Autodesk Inventor part; units mm, degrees
ref_plane "Work Plane1" through (29, 0, 0) normal (0, -1, 0) x (1, 0, 0)
ref_plane "YZ Plane" through (0, 0, 0) normal (1, 0, 0) x (0, 1, 0)
ref_plane "XZ Plane" through (0, 0, 0) normal (0, 1, 0) x (-1, 0, 0)
sketch "Sketch1" plane through (0, 0, 0) normal (0, 0, 1) x (1, 0, 0)
  line L0 (-2.6667, 0) -> (20, 0)
  line L1 (20, 0) -> (20, 6)
  line L2 (20, 6) -> (4.375, 6)
  line L3 (4.375, 6) -> (3.3014, 6)
  line L4 (3.3014, 6) -> (0, 6)
  line L5 (0, 6) -> (0, 9)
  line L6 (0, 9) -> (-12, 9)
  line L7 (-12, 9) -> (-12, 5.7735)
  line L8 (-12, 5.7735) -> (-6, 5.7735)
  line L9 (-6, 5.7735) -> (-2.6667, 0)
  line L10 (-18.4, 0) -> (26.4, 0)
  line L11 (0, -1.8) -> (0, 10.8)
  line L12 (4.375, 6) -> (0, 6) construction
  dimension "d1" = 15.625
  dimension "d2" = 1.0736
  dimension "d3" = 12
  dimension "d4" = 6
  dimension "d5" = 60
  dimension "d6" = 12
  dimension "d7" = 12
  dimension "d8" = 11.547
  dimension "d9" = 18
  dimension "d26" = 20
revolve "Body" add sketch "Sketch1" angle 360 about axis through (-2.6667, 0, 0) along (1, 0, 0)
sketch "Sketch2" plane through (-12, 0, 0) normal (-1, 0, 0) x (0, 0, 1)
  circle A0 centre (0, 0) radius 5.7735
  line L0 (0, -12.6) -> (0, 12.6)
  line L1 (-12.6, 0) -> (12.6, 0)
  line L2 (5.7735, 0) -> (2.8868, -5)
  line L3 (2.8868, -5) -> (-2.8868, -5)
  line L4 (-2.8868, -5) -> (-5.7735, 0)
  line L5 (-5.7735, 0) -> (-2.8868, 5)
  line L6 (-2.8868, 5) -> (2.8868, 5)
  line L7 (2.8868, 5) -> (5.7735, 0)
extrude "Slot" add sketch "Sketch2" against normal up to next contours L7 A0 | A0 L2 | L6 L0 A0 | A0 L0 L3 | L0 L6 A0 | A0 L3 L0 | L4 A0 | A0 L5
fillet "Fillet1" radius 1.2 1 edges at (-12, -9, 0)
thread "Thread"
chamfer "Chamfer1" distance 1.0735 distance2 1.0735 1 edges at (20, -6, 0) measured on face at (20, -3.0269, -1.5886)
ref_plane "Work Plane1" through (29, 0, 0) normal (0, -1, 0) x (1, 0, 0)
fillet "Fillet2" radius 0.1 1 edges at (0, -6, 0)
equation "\"d1\" = GEL"
equation "\"d3\" = KOH"
equation "\"d4\" = INTI"
equation "\"d6\" = GD"
equation "\"d7\" = BDM"
equation "\"d8\" = 1.1547 * SW"
equation "\"d9\" = KOD"
equation "\"d26\" = NLG"
equation "\"d30\" = R"
equation "\"d17\" = RR"
equation "\"d13\" = GEL"
equation "\"d15\" = -0.5 * SPD + 0.5 * GD"
equation "\"d16\" = GUL"
equation "\"GD\" = NND"
equation "\"NLG\" = 20"
equation "\"GEL\" = 15.625"
equation "\"KOD\" = 18"
equation "\"KOH\" = NND"
equation "\"INTI\" = 6"
equation "\"GAL\" = 0.61345 * PTC"
equation "\"GUL\" = 0.61345 * PTC"
equation "\"BDM\" = NND"
equation "\"RR\" = 0.1 * NND"
equation "\"SPD\" = NND - 1.2269 * PTC"
equation "\"R\" = 0.1"
equation "\"PHH\" = 0.25"
equation "\"GD1\" = THREADDIA - 1.2269 * PTC"
equation "\"THREADDIA\" = 12"
equation "\"FAWI\" = 45deg"
equation "\"PTC\" = 1.75"
equation "\"KOH1\" = 10.8"
equation "\"NND\" = 12"
equation "\"TOA\" = 30deg"
equation "\"E0\" = 1.155 * SW"
properties part number "AS 1420 - 1973 - M12 x 20" material "Steel, Mild"
Geometry check sheet. Reference: the model listing, model coordinates, mm. A direction names the side the tool comes from. Coordinates: 2 decimals unless noted, no trailing zeros. Order: outer loops, then holes, each group sorted by start corner. A loop starts at its lowest first (then second) coordinate and runs counter-clockwise, first axis right, second up. Notation, with made-up numbers: (54, -10) -> (111, -10) arc R15 cw to (111, 18) -> close; hole circle Ø10 at (70.25, 66). An arc over 180 degrees is marked (long way). Use a Markdown table: item, result. Add a question column.
1. Cross-section at A-A (x = 13). Enter the section's corners in (y, z), and give its area (3 significant figures).
2. Set-up check for faces 4 (the face through (20, 0, 0)), 5 (the face through (-9, 5, 0)): record each of +Z, -Z, +X, -X, +Y, -Y from which the full face is reachable in a straight line by a thin tool's end or side.
3. Material ranges on L1, parallel to X at y = -4.75, z = 5.5; L2, parallel to Z at x = -3, y = 0.25; L3, parallel to Z at x = -4, y = 0.25, recorded low to high.
4. Go/stop test with flat-tipped pins: pin 1 Ø10 at (x, z) = (-6, -4) entering from +Y; pin 2 Ø5 at (y, z) = (6, 5.5) entering from +X; pin 3 Ø1.5 at (y, z) = (7, -5.5) entering from -X; pin 4 Ø10 at (x, y) = (7, 0.5) entering from -Z. Record where each tip stops, or that it passes through.
5. Mould release check, pull along Z, two halves, no side actions. Record for faces 1 (the face through (9, -6, 0)), 2 (the face through (0, 2, -6)), 3 (the face through (-8.822, -2.465, 4.35)): pulls with the +Z half, pulls with the -Z half, needs draft (parallel to the pull), parting line crosses it, or undercut.
Filled sheet:
| question | item | result |
|---|---|---|
| 1 | outline | circle Ø12 at (0, 0) |
| 1 | area | 113 mm2 |
| 2 | face 4 | +Z, -Z, +X, +Y, -Y |
| 2 | face 5 | -X |
| 3 | L1 | -12 to 0 |
| 3 | L2 | -9 to -0.52, 0.52 to 9 |
| 3 | L3 | -9 to -2.3, 2.3 to 9 |
| 4 | pin 1 | y = 9 |
| 4 | pin 2 | x = 19.29 |
| 4 | pin 3 | x = -11.95 |
| 4 | pin 4 | z = -6 |
| 5 | face 1 | parting line crosses it |
| 5 | face 2 | needs draft |
| 5 | face 3 | undercut |
